Could you check a few things on this model? Use its own coordinates, in mm. A direction names the side the tool comes from. Round coordinates to 2 decimals unless told otherwise and drop trailing zeros. Loops run counter-clockwise (first coordinate to the right, second up) from the corner with the lowest first, then second, coordinate; pieces in that order, holes last.
from build123d import *

# Parameters (mm, degrees)
SKETCH_1_W      = 26.990014613
SKETCH_1_H      = 7
M10X1_251_D     = 8.8
M10X1_251_DEPTH = 26.25
M10X1_251_TIP   = 2.643786724


with BuildPart() as part:
    # Эскиз1 → Повернуть1 (revolve)
    with BuildSketch(Plane(origin=(0, 0, 0), x_dir=(0, 0, -1), z_dir=(1, 0, 0))):
        with Locations((-13.495007307, 3.5)):
            Rectangle(SKETCH_1_W, SKETCH_1_H)
    revolve(axis=Axis((0, 0, 1000), (0, 0, -1)))

    # Отверстие обработанное метчиком M10x1.251
    with Locations(Plane.XY.offset(26.990014613)):
        with Locations((0, 0)):
            Hole(M10X1_251_D / 2, depth=M10X1_251_DEPTH)
            with Locations((0, 0, -(M10X1_251_DEPTH + M10X1_251_TIP / 2))):  # 118° drill point
                Cone(0, M10X1_251_D / 2, M10X1_251_TIP, mode=Mode.SUBTRACT)

    # Зеркальное отражение1: part across plane


with BuildPart() as part_1:
    add(part.part)
    add(part.part.mirror(Plane.XY))


solid = part_1.part
Item 1: We'd pull the mould along X, two halves only. Please class faces 1 (the flat face through (-5, 0, 26.99)), 2 (the cylindrical face through (-4.197, 1.322, -13.681)): released by +X, released by -X, zero draft, split by the parting line, or undercut.
Results list:
face 1: zero draft
face 2: undercut
Item 2: Will these pins go through, and if not, where does the flat tip stop? pin 1 (8 mm diameter, centred on x = 0, y = 0, fed in from +Z); pin 2 (1 mm diameter, centred on x = -3, z = -18, fed in from -Y); pin 3 (2 mm diameter, centred on x = -2, z = 12.5, fed in from -Y).
Results list:
pin 1: stops at z = 0.5
pin 2: stops at y = -6.54
pin 3: stops at y = -6.93
Item 3: If we section it at D-D, the plane y = -5: Please give me the cut outline in (x, z), then the cut area to 3 significant figures.
Results list:
outline: (-4.9, -26.99) - (4.9, -26.99) - (4.9, 26.99) - (-4.9, 26.99) - close
area: 529 mm2
Item 4: If we section it at A-A, the plane x = 0: Please give me the cut outline in (y, z), then the cut area to 3 significant figures.
Results list:
outline: (-7, -26.99) - (-4.4, -26.99) - (-4.4, -0.74) - (-3.17, 0) - (-4.4, 0.74) - (-4.4, 26.99) - (-7, 26.99) - close; (3.17, 0) - (4.4, -0.74) - (4.4, -26.99) - (7, -26.99) - (7, 26.99) - (4.4, 26.99) - (4.4, 0.74) - close
area: 283 mm2
Item 5: If I drill on line 1 along X through (y, z) = (0, -20); line 2 along X through (y, z) = (3.25, -21); line 3 along Y through (x, z) = (-2.5, -5.5), over which ranges is the centre line in solid material (lowest first)?
Results list:
line 1: x = -7 to -4.4, 4.4 to 7
line 2: x = -6.2 to -2.97, 2.97 to 6.2
line 3: y = -6.54 to -3.62, 3.62 to 6.54
Item 6: If we section it at C-C, the plane z = -18: Please give me the cut outline in (x, y).
Results list:
outline: circle Ø14 at (0, 0); hole circle Ø8.8 at (0, 0)
Item 7: For faces 3 (the cylindrical face through (-4.197, 1.322, 13.681)), 4 (the flat face through (-5, 0, -26.99)), which set-ups out of +Z, -Z, +X, -X, +Y, -Y let a thin tool reach every point of the face, with its end or its side?
Results list:
face 3: +Z
face 4: -Z, +X, -X, +Y, -Y
